CAD build for the part. Positions are in the model's coordinates, mm. Face numbers are marked on the shaded views. A direction names the side the tool comes from. Round coordinates to 2 decimals unless told otherwise and drop trailing zeros. Loops run counter-clockwise (first coordinate to the right, second up) from the corner with the lowest first, then second, coordinate; pieces in that order, holes last. Notation, with made-up numbers: (50, -40) - (86, -40) arc R22 cw to (86, -29) - close; hole circle Ø2 at (23, 12). An arc over 180 degrees is marked (long way). One line per question, with ' | ' between items.
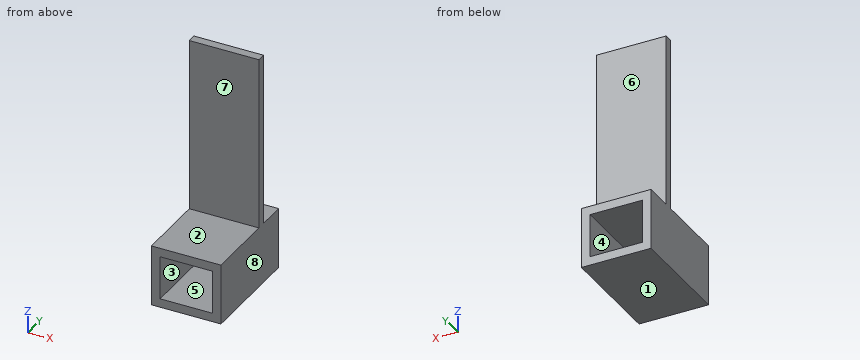
```python
from build123d import *

# Parameters (mm, degrees)
SKETCH_1_W      = 12
SKETCH_1_H      = 10
EXTRUDE_1_DEPTH = 25
SHELL_1_T       = 2
SKETCH_2_W      = 16
SKETCH_2_H      = 2.007499683
EXTRUDE_2_DEPTH = 40


with BuildPart() as part:
    # 草图1 → 凸台-拉伸1 (new body)
    with BuildSketch(Plane(origin=(0, 0, 0), x_dir=(1, 0, 0), z_dir=(0, 1, 0))):
        with Locations((6, -5)):
            Rectangle(SKETCH_1_W, SKETCH_1_H)
    extrude(amount=EXTRUDE_1_DEPTH)

    # 抽壳1
    shell_1_openings = [part.faces().sort_by_distance(p)[0] for p in [
        (6, 0, 5),
        (6, 25, 5),
    ]]
    offset(amount=SHELL_1_T, openings=shell_1_openings, kind=Kind.INTERSECTION)

    # 草图2 → 凸台-拉伸2 (add)
    with BuildSketch(Plane.XY.offset(12)):
        with Locations((6, 17.450698372)):
            Rectangle(SKETCH_2_W, SKETCH_2_H)
    extrude(amount=EXTRUDE_2_DEPTH)


solid = part.part
```
(1) Probe L1, parallel to Z at x = 10.25, y = 21.75; L2, parallel to X at y = 2, z = 1.5; L3, parallel to Y at x = 10.75, z = 41. List the from-to ranges inside material, lowest first.
Results found:
L1: z = -2 to 0, 10 to 12 | L2: x = -2 to 0, 12 to 14 | L3: y = 16.45 to 18.45
(2) Cut at B-B, the plane y = 9. Write the cut outline in (x, z), then the cut area to 3 significant figures.
Results found:
outline: (-2, -2) - (14, -2) - (14, 12) - (-2, 12) - close; hole (0, 0) - (12, 0) - (12, 10) - (0, 10) - close | area: 104 mm²
(3) Tool access for the marked faces 5, 6, 7 and 8: list every direction of +Z, -Z, +X, -X, +Y, -Y with a clear straight run to the whole face (end or side of a thin tool).
Results found:
face 5: +Y, -Y | face 6: +Z, +X, -X, +Y | face 7: +Z, +X, -X, -Y | face 8: +Z, -Z, +X, +Y, -Y
(4) Cut at A-A, the plane x = 10.25. Write the cut outline in (y, z).
Results found:
outline: (0, -2) - (25, -2) - (25, 0) - (0, 0) - close; (0, 10) - (25, 10) - (25, 12) - (18.45, 12) - (18.45, 52) - (16.45, 52) - (16.45, 12) - (0, 12) - close
(5) Two-plate mould, pull along Z, no slides. Class the marked faces 1, 2, 3 and 4: released by +Z, released by -Z, zero draft, split by the parting line, or undercut.
Results found:
face 1: released by -Z | face 2: released by +Z | face 3: undercut | face 4: undercut
(6) Drop flat-ended pins along their axis: P1, Ø1, axis at x = 9.5, z = 19.5, coming from the -Y side; P2, Ø9.5, axis at x = 7, y = 9, coming from the +Z side; P3, Ø1.5, axis at x = 9.5, z = 15, coming from the +Y side. Give the stop position or say it passes through.
Results found:
P1: stops at y = 16.45 | P2: stops at z = 12 | P3: stops at y = 18.45
(7) Cut at C-C, the plane z = 21. Write the cut outline in (x, y), then the cut area to 3 significant figures.
Results found:
outline: (-2, 16.45) - (14, 16.45) - (14, 18.45) - (-2, 18.45) - close | area: 32.1 mm²
